Input: part model. Units: mm. Frame: model coordinates. Face numbers are marked on the shaded views. Give positions to 0.01 mm unless a question says otherwise; leave off trailing zeros. Loops run counter-clockwise (first coordinate to the right, second up) from the corner with the lowest first, then second, coordinate; pieces in that order, holes last. Notation, with made-up numbers: (-26.75, -38.5) - (-0.75, -38.5) arc R17 ccw to (-0.75, -13.5) - close; hole circle Ø2 at (19, -27.75). An arc over 180 degrees is marked (long way). Answer as a JSON object with one key per item and string values.
from build123d import *

# Parameters (mm, degrees)
F0_R     = 60
F0_R_2   = 3
F0_R_3   = 15
F1_DEPTH = 30


with BuildPart() as f1:
    # F0 (on Front) → F1 (new body)
    with BuildSketch(Plane.XZ):
        Circle(F0_R)
        with Locations((-35.401378, -33.233948)):
            Circle(F0_R_2, mode=Mode.SUBTRACT)
        with BuildLine():
            Line((-12.483101, -19.940369), (10.516899, -19.940369))
            ThreePointArc((10.516899, -19.940369), (13.523289, -20.747911), (15.720417, -22.953163))
            Line((15.720417, -22.953163), (21.751998, -33.459784))
            ThreePointArc((21.751998, -33.459784), (22.51142, -35.781151), (22.282739, -38.212853))
            ThreePointArc((22.282739, -38.212853), (-1.895302, -56.274409), (-26.469163, -38.755197))
            ThreePointArc((-26.469163, -38.755197), (-26.694895, -35.88137), (-25.554285, -33.233948))
            Line((-25.554285, -33.233948), (-17.261779, -22.312113))
            ThreePointArc((-17.261779, -22.312113), (-15.150541, -20.565914), (-12.483101, -19.940369))
        make_face(mode=Mode.SUBTRACT)
        with BuildLine():
            ThreePointArc((-25.57569, 0), (-17.203021, -4.661994), (-22.39679, -12.715598))
            Line((-22.39679, -12.715598), (-38.002294, -26.009176))
            ThreePointArc((-38.002294, -26.009176), (-53.620423, -21.803036), (-47.250003, -6.93578))
            Line((-47.250003, -6.93578), (-25.57569, 0))
        make_face(mode=Mode.SUBTRACT)
        with Locations((33.667434, -34.678902)):
            Circle(F0_R_2, mode=Mode.SUBTRACT)
        with BuildLine():
            ThreePointArc((16.327983, -17.05046), (15.252019, -11.740154), (20.662844, -11.457273))
            Line((20.662844, -11.457273), (44.998671, -13.827356))
            ThreePointArc((44.998671, -13.827356), (48.186477, -25.295435), (36.723992, -28.503295))
            Line((36.723992, -28.503295), (16.327983, -17.05046))
        make_face(mode=Mode.SUBTRACT)
        with Locations((46.383031, -6.068808)):
            Circle(F0_R_2, mode=Mode.SUBTRACT)
        with Locations((-51.873855, 0)):
            Circle(F0_R_2, mode=Mode.SUBTRACT)
        with BuildLine():
            Line((-18.010051, 14.654659), (-20.884113, 10.975861))
            ThreePointArc((-20.884113, 10.975861), (-22.981972, 9.27699), (-25.612258, 8.669726))
            Line((-25.612258, 8.669726), (-41.092021, 8.669726))
            ThreePointArc((-41.092021, 8.669726), (-44.989315, 10.107807), (-47.0184, 13.732693))
            ThreePointArc((-47.0184, 13.732693), (-43.773022, 28.201746), (-31.494693, 36.516107))
            ThreePointArc((-31.494693, 36.516107), (-27.83933, 36.174602), (-25.067187, 33.767627))
            Line((-25.067187, 33.767627), (-17.60701, 21.458334))
            ThreePointArc((-17.60701, 21.458334), (-16.748697, 17.993713), (-18.010051, 14.654659))
        make_face(mode=Mode.SUBTRACT)
        with Locations((-20.662844, 42.966518)):
            Circle(F0_R_2, mode=Mode.SUBTRACT)
        Circle(F0_R_3, mode=Mode.SUBTRACT)
        with BuildLine():
            ThreePointArc((18.963135, 11.921459), (16.459409, 15.771092), (17.41111, 20.263594))
            Line((17.41111, 20.263594), (22.259295, 27.328092))
            ThreePointArc((22.259295, 27.328092), (24.762361, 29.412708), (27.985799, 29.882196))
            ThreePointArc((27.985799, 29.882196), (42.683104, 21.611507), (47.564314, 5.468741))
            ThreePointArc((47.564314, 5.468741), (45.63834, 1.573514), (41.58788, 0))
            Line((41.58788, 0), (28.101831, 0))
            ThreePointArc((28.101831, 0), (23.859191, 1.757359), (22.101831, 6))
            Line((22.101831, 6), (22.101831, 6.608079))
            ThreePointArc((22.101831, 6.608079), (21.410802, 9.403581), (19.496887, 11.555159))
            Line((19.496887, 11.555159), (18.963135, 11.921459))
        make_face(mode=Mode.SUBTRACT)
        with BuildLine():
            Line((12.861297, 42.56715), (7.310784, 20.229358))
            ThreePointArc((7.310784, 20.229358), (0.050757, 17.019958), (-7.209271, 20.229358))
            Line((-7.209271, 20.229358), (-11.240784, 42.966518))
            ThreePointArc((-11.240784, 42.966518), (-9.931036, 47.868572), (-5.332932, 50.014036))
            Line((-5.332932, 50.014036), (7.038366, 50.014036))
            ThreePointArc((7.038366, 50.014036), (11.764957, 47.709891), (12.861297, 42.56715))
        make_face(mode=Mode.SUBTRACT)
        with Locations((22.107799, 42.56715)):
            Circle(F0_R_2, mode=Mode.SUBTRACT)
    extrude(amount=F1_DEPTH)


solid = f1.part
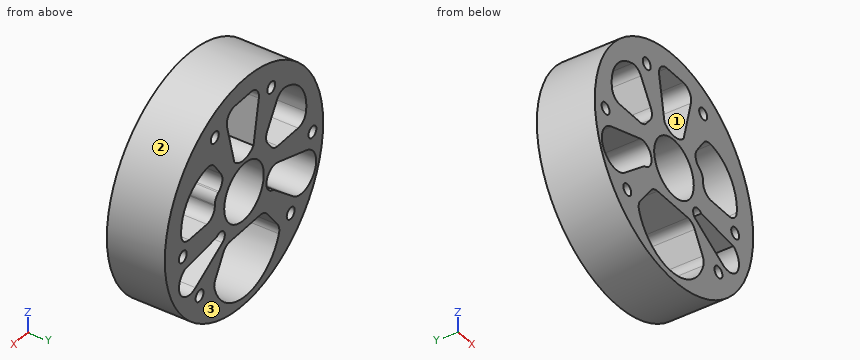
Item 1: Cut plane A-A (x = -44.5). Return loops of the section in (y, z).
Geometry check:
{"outline": "(-30, -40.25) - (0, -40.25) - (0, -27.83) - (-30, -27.83) - close; (-30, -6.06) - (0, -6.06) - (0, 9.73) - (-30, 9.73) - close; (-30, 27.05) - (0, 27.05) - (0, 40.25) - (-30, 40.25) - close"}
Item 2: Contact query for flat-ended pins moving along their axis: P1, Ø5.5, axis at x = -20.66, z = 42.97, coming from the -Y side; P2, Ø3.5, axis at x = 2, y = -19.5, coming from the -Z side; P3, Ø6, axis at x = -47.5, y = -5, coming from the -Z side; P4, Ø17, axis at x = -29.5, y = -17, coming from the +Z side (3 decimals). Output: stop coordinate, or through.
Geometry check:
{"P1": "passes through", "P2": "stops at z = -60", "P3": "stops at z = -40.25", "P4": "stops at z = 56.205"}
Item 3: Cut plane B-B (x = 0). Return loops of the section in (y, z), then the cut area to 3 significant figures.
Geometry check:
{"outline": "(-30, -60) - (0, -60) - (0, -56.18) - (-30, -56.18) - close; (-30, -19.94) - (0, -19.94) - (0, -15) - (-30, -15) - close; (-30, 15) - (0, 15) - (0, 17.02) - (-30, 17.02) - close; (-30, 50.01) - (0, 50.01) - (0, 60) - (-30, 60) - close", "area": "623 mm2"}
Item 4: Mould query, pull axis X, two halves, no side actions, for the marked faces 1, 2 and 3. Classes: released by +X, released by -X, zero draft, split by the parting line, or undercut.
Geometry check:
{"face 1": "undercut", "face 2": "split by the parting line", "face 3": "zero draft"}
Item 5: Cut plane C-C (y = -10.5). Give the number of separate pieces and of enclosed holes in the cut face, then the cut area to 3 significant figures.
Geometry check:
{"separate pieces": "1", "enclosed holes": "13", "area": "6,000 mm2"}
Item 6: Material intervals for line 1 (X direction, y = -5.75, z = -11); line 2 (Z direction, x = 17, y = -27.5); line 3 (Z direction, x = -13, y = -13.5), sorted ascending. Write a range as [from, to].
Geometry check:
{"line 1": "x = [-58.98, -52.76], [-19.03, -10.2], [10.2, 16.03], [20.13, 58.98]", "line 2": "z = [-57.54, -47.63], [-25.18, -17.43], [-10.52, 14.17], [19.57, 57.54]", "line 3": "z = [-58.57, -53.88], [-19.96, -7.48], [7.48, 58.57]"}
